from build123d import *

# Parameters (mm, degrees)
SKETCH2_W           = 33.887326606
SKETCH2_H           = 19.760086797
BOSS_EXTRUDE1_DEPTH = 15
SKETCH3_W           = 33.887326606
SKETCH3_H           = 19.760086797
BOSS_EXTRUDE2_DEPTH = 2
SKETCH6_W           = 32
SKETCH6_H           = 34.760086797
SKETCH6_R           = 2
BOSS_EXTRUDE4_DEPTH = 2.624753
FILLET1_R           = 4


with BuildPart() as part:
    # Sketch2 → Boss-Extrude1 (new body)
    with BuildSketch(Plane.XY):
        with Locations((0, -7.586628603)):
            Rectangle(SKETCH2_W, SKETCH2_H)
        with BuildLine():
            Line((0, 0), (14.318912319, -14.318912319))
            Line((14.318912319, -14.318912319), (12.833988079, -15.80383656))
            Line((12.833988079, -15.80383656), (1.060660172, -4.030508653))
            ThreePointArc((1.060660172, -4.030508653), (0, -3.591168825), (-1.060660172, -4.030508653))
            Line((-1.060660172, -4.030508653), (-12.833988079, -15.80383656))
            Line((-12.833988079, -15.80383656), (-14.318912319, -14.318912319))
            Line((-14.318912319, -14.318912319), (0, 0))
        make_face(mode=Mode.SUBTRACT)
    extrude(amount=BOSS_EXTRUDE1_DEPTH)

    # Sketch3 → Boss-Extrude2 (add)
    with BuildSketch(Plane.XY.offset(15)):
        with Locations((0, -7.586628603)):
            Rectangle(SKETCH3_W, SKETCH3_H)
    extrude(amount=BOSS_EXTRUDE2_DEPTH)

    # Sketch6 → Boss-Extrude4 (add)
    with BuildSketch(Plane(origin=(16.943663303, 0, 0), x_dir=(0, 0, -1), z_dir=(1, 0, 0))):
        with Locations((-16, -15.086628602)):
            Rectangle(SKETCH6_W, SKETCH6_H)
        with Locations((-8.5, -27.466672001)):
            Circle(SKETCH6_R, mode=Mode.SUBTRACT)
        with Locations((-27, -27.466672001)):
            Circle(SKETCH6_R, mode=Mode.SUBTRACT)
        with Locations((-27, -2.706585204)):
            Circle(SKETCH6_R, mode=Mode.SUBTRACT)
    extrude(amount=-BOSS_EXTRUDE4_DEPTH)

    # Fillet1
    fillet1_edges = [part.edges().sort_by_distance(p)[0] for p in [
        (14.318910303, -7.586628602, 17),
        (14.318910303, -17.466672001, 8.5),
    ]]
    fillet(fillet1_edges, radius=FILLET1_R)


solid = part.part
Can you work these out from the model? Positions are in its coordinate system, mm. A direction names the side the tool comes from. Coordinates: 2 decimals unless noted, no trailing zeros. Write each loop counter-clockwise with the first axis right and the second up, starting at its lowest first coordinate (ties: lowest second). Pieces come first, ordered by that corner, then holes. Notation, with made-up numbers: (77.25, -23) -> (89.25, -23) arc R3 ccw to (89.25, -19) -> close; hole circle Ø4 at (56, -37.5). An arc over 180 degrees is marked (long way). Write item = value, one per line.
(1) For pin 1 (5 mm diameter, centred on y = -27.47, z = 8.5, fed in from -X); pin 2 (8 mm diameter, centred on x = 3, z = 13, fed in from -Y); pin 3 (10 mm diameter, centred on x = -2.5, y = -5.5, fed in from +Z), each with a flat end and sliding along its axis, tell me the tip position at first contact or that it passes through.
Verdict:
pin_1 = 14.32
pin_2 = -17.47
pin_3 = 17
(2) Imagine slicing it at B-B (z = 8.5). State how many separate pieces and enclosed holes the cut face has, and give its area (3 significant figures).
Verdict:
separate_pieces = 2
enclosed_holes = 1
area = 621 mm^2
(3) If I drill on probe 1 along Y at (x, z) = (16.2, 27); probe 2 along Y at (x, z) = (15.75, 8.5); probe 3 along Z at (x, y) = (6, -17), over which ranges is the centre line in solid material (lowest first)?
Verdict:
probe_1 = -32.47 to -29.47, -25.47 to -4.71, -0.71 to 2.29
probe_2 = -32.47 to -29.47, -25.47 to 2.29
probe_3 = 0 to 17
(4) Imagine slicing it at C-C (y = -28). Please give me the cut outline in (x, z).
Verdict:
outline = (14.32, 0) -> (16.94, 0) -> (16.94, 6.57) -> (14.32, 6.57) -> close; (14.32, 10.43) -> (16.94, 10.43) -> (16.94, 25.07) -> (14.32, 25.07) -> close; (14.32, 28.93) -> (16.94, 28.93) -> (16.94, 32) -> (14.32, 32) -> close
(5) Imagine slicing it at A-A (z = 27). Please give me the cut outline in (x, y).
Verdict:
outline = (14.32, -32.47) -> (16.94, -32.47) -> (16.94, -29.47) -> (14.32, -29.47) -> close; (14.32, -25.47) -> (16.94, -25.47) -> (16.94, -4.71) -> (14.32, -4.71) -> close; (14.32, -0.71) -> (16.94, -0.71) -> (16.94, 2.29) -> (14.32, 2.29) -> close
(6) Thinking about a two-plate mould opening in Z: for faces 1 (the face through (15.65, -29.241, 26.077)), 2 (the face through (15.65, -29.42, 8.93)), 3 (the face through (16.944, -15, 16)), 4 (the face through (-4, -7, 17)), which applies, +Z half, -Z half, draft (parallel to the pull), parting line (faces both ways), or undercut?
Verdict:
face_1 = undercut
face_2 = undercut
face_3 = draft
face_4 = +Z half
(7) On a 3-axis mill with a long thin cutter (end or side, diameter ignored), from which of +Z, -Z, +X, -X, +Y, -Y can I reach the whole of each face in a straight line? I mean faces 5 (the face through (-16.944, -8, 8)), 6 (the face through (0, -8, 0)), 7 (the face through (14.319, -19, 23)), 8 (the face through (-4, -17.467, 8)), 9 (the face through (-6.86, -9.83, 7.4)). Say none if no direction works.
Verdict:
face_5 = +Z, -Z, -X, +Y, -Y
face_6 = -Z, +X, -X, +Y, -Y
face_7 = +Z, -X, -Y
face_8 = +Z, -Z, -X, -Y
face_9 = -Z
